Autodesk Inventor part; units mm, degrees
ref_plane "b_s_XY" through (0, 38, 5) normal (0, 1, 0) x (1, 0, 0)
ref_plane "b_s_YZ" through (0, 38, 5) normal (1, 0, 0) x (0, 0, -1)
ref_plane "b_s_ZX" through (0, 38, 5) normal (0, 0, -1) x (0, 1, 0)
sketch "Sketch_9" plane through (0, 0, 0) normal (0, 0, 1) x (1, 0, 0)
  line L0 (-15, 5) -> (-15, 0)
  line L1 (-15, 0) -> (15, 0)
  line L2 (15, 0) -> (15, 5)
  arc A0 (15, 5) -> (14, 6) centre (14, 5) ccw
  line L3 (14, 6) -> (-14, 6)
  arc A1 (-14, 6) -> (-15, 5) centre (-14, 5) ccw
sketch "Sketch_10" plane through (0, 0, 0) normal (0, 1, 0) x (-1, 0, 0)
  line L0 (15, 1) -> (15, 9)
  arc A0 (15, 9) -> (14, 10) centre (14, 9) ccw
  line L1 (14, 10) -> (-14, 10)
  arc A1 (-14, 10) -> (-15, 9) centre (-14, 9) ccw
  line L2 (-15, 9) -> (-15, 1)
  arc A2 (-15, 1) -> (-14, 0) centre (-14, 1) ccw
  line L3 (-14, 0) -> (14, 0)
  arc A3 (14, 0) -> (15, 1) centre (14, 1) ccw
extrude "Extrusion1" add sketch "Sketch_9" along normal blind 20
extrude "Extrusion2" add sketch "Sketch_10" along normal blind 38
sketch "Sketch_5" plane through (0, 0, 0) normal (0, 0, 1) x (1, 0, 0)
  arc A0 (-14, 38) -> (-15, 37) centre (-14, 37) ccw
  line L0 (-14, 38) -> (14, 38)
  arc A1 (15, 37) -> (14, 38) centre (14, 37) ccw
  line L1 (15, 37) -> (15, 76)
  line L2 (15, 76) -> (-15, 76)
  line L3 (-15, 76) -> (-15, 37)
extrude "Extrusion3" cut sketch "Sketch_5" along normal blind 10
sketch "Sketch_7" plane through (0, 0, 0) normal (1, 0, 0) x (0, 1, 0)
  line L0 (25, 0) -> (25, 10)
  line L1 (25, 10) -> (34, 10)
  line L2 (34, 10) -> (33, 9)
  line L3 (33, 9) -> (33, 1)
  line L4 (33, 1) -> (34, 0)
  line L5 (34, 0) -> (25, 0)
  line L6 (25, 0) -> (25, 10)
revolve "Revolution1" cut sketch "Sketch_7" angle 360 about axis through (0, 25, 0) along (0, 0, -1)
sketch "Sketch_1" plane through (0, 0, 5) normal (0, 0, 1) x (1, 0, 0)
  line L0 (0, 25) -> (0, 38)
  line L1 (0, 38) -> (2, 38)
  line L2 (2, 38) -> (1.621, 37.621)
  line L3 (1.621, 37.621) -> (1.621, 33)
  line L4 (1.621, 33) -> (2, 32.621)
  line L5 (2, 32.621) -> (2, 25)
  line L6 (2, 25) -> (0, 25)
  line L7 (0, 25) -> (0, 38)
revolve "Revolution2" cut sketch "Sketch_1" angle 360 about axis through (0, 25, 5) along (0, -1, 0)
thread "Thread1"
sketch "Sketch6" plane through (-14, 6, 20) normal (0, 1, 0) x (1, 0, 0)
  point P0 (7.5, 5)
hole "Hole1" at (-6.5, 6, 15) direction (0, -1, 0) diameter 5.5 depth 6 countersink diameter 6.5 countersink angle 90
sketch "Sketch7" plane through (-14, 6, 20) normal (0, 1, 0) x (1, 0, 0)
  point P0 (20.5, 5)
hole "Hole2" at (6.5, 6, 15) direction (0, -1, 0) diameter 5.5 depth 6 countersink diameter 6.5 countersink angle 90
sketch "Sketch_4" plane through (0, 0, 0) normal (0, 1, 0) x (-1, 0, 0)
  line L0 (30, -10) -> (30, 30)
  line L1 (30, 30) -> (-30, 30)
  line L2 (-30, 30) -> (-30, -10)
  line L3 (-30, -10) -> (30, -10)
  line L4 (15, 1) -> (15, 19)
  arc A0 (15, 19) -> (14, 20) centre (14, 19) ccw
  line L5 (14, 20) -> (-14, 20)
  arc A1 (-14, 20) -> (-15, 19) centre (-14, 19) ccw
  line L6 (-15, 19) -> (-15, 1)
  arc A2 (-15, 1) -> (-14, 0) centre (-14, 1) ccw
  line L7 (-14, 0) -> (14, 0)
  arc A3 (14, 0) -> (15, 1) centre (14, 1) ccw
extrude "Extrusion4" cut sketch "Sketch_4" along normal blind 38
sketch "Sketch_8" plane through (0, 0, 0) normal (0, 0, 1) x (1, 0, 0)
  line L0 (-7, 10) -> (-7, 2)
  line L1 (-7, 2) -> (7, 2)
  line L2 (7, 2) -> (7, 10)
  line L3 (7, 10) -> (-7, 10)
extrude "Extrusion5" cut sketch "Sketch_8" along normal blind 0.8
sketch "Sketch_6" plane through (0, 0, 0) normal (1, 0, 0) x (0, 1, 0)
  line L0 (57, 30) -> (-19, 30)
  line L1 (-19, 30) -> (-19, -10)
  line L2 (-19, -10) -> (57, -10)
  line L3 (57, -10) -> (57, 30)
  line L4 (5, 20) -> (0, 20)
  line L5 (0, 20) -> (0, 0)
  line L6 (0, 0) -> (37, 0)
  arc A0 (37, 0) -> (38, 1) centre (37, 1) ccw
  line L7 (38, 1) -> (38, 9)
  arc A1 (38, 9) -> (37, 10) centre (37, 9) ccw
  line L8 (37, 10) -> (6, 10)
  line L9 (6, 10) -> (6, 19)
  arc A2 (6, 19) -> (5, 20) centre (5, 19) ccw
extrude "Extrusion6" cut sketch "Sketch_6" along normal mid plane 30
sketch "Sketch_11" plane through (0, 0, 0) normal (1, 0, 0) x (0, 1, 0)
  line L0 (6, 11) -> (3, 11)
  line L1 (3, 11) -> (3, 5)
  line L2 (3, 5) -> (7, 5)
  line L3 (7, 5) -> (7, 10)
  arc A0 (6, 11) -> (7, 10) centre (7, 11) ccw
extrude "Extrusion7" add sketch "Sketch_11" along normal mid plane 28
ref_plane "b_s_XY" through (0, 38, 5) normal (0, 1, 0) x (1, 0, 0)
ref_plane "b_s_YZ" through (0, 38, 5) normal (1, 0, 0) x (0, 0, -1)
ref_plane "b_s_ZX" through (0, 38, 5) normal (0, 0, -1) x (0, 1, 0)
properties part number "SHKLMT16b"
The model under review builds one solid part; all positions refer to its coordinate system, in mm. A direction names the side the tool comes from. Coordinates: 2 decimals unless noted, no trailing zeros. Order: outer loops, then holes, each group sorted by start corner. A loop starts at its lowest first (then second) coordinate and runs counter-clockwise, first axis right, second up. Notation, with made-up numbers: (-33, 81.25) -> (-8, 81.25) arc R21 ccw to (-8, 87.25) -> close; hole circle Ø7 at (7, 0). An arc over 180 degrees is marked (long way). Answer in a Markdown table with one row per item.
(1) Insertion check: pin 1 (9 mm diameter, centred on x = -0.5, y = 6.5, fed in from -Z); pin 2 (5 mm diameter, centred on x = -6.5, z = 15, fed in from +Y); pin 3 (0.8 mm diameter, centred on y = 6.5, z = 10.5, fed in from +X); pin 4 (14 mm diameter, centred on x = 0, y = 17, fed in from +Z). Each pin has a flat end and moves straight along its axis. Give the tip position at first contact, or say it passes through.
Answers:
| item | result |
|---|---|
| pin 1 | z = 0 |
| pin 2 | through |
| pin 3 | x = 14 |
| pin 4 | z = 10 |
(2) Consider section D-D (z = 5). Write out the cut boundary in (x, y), plus the area to 3 significant figures.
Answers:
| item | result |
|---|---|
| outline | (-15, 0) -> (15, 0) -> (15, 37) arc R1 ccw to (14, 38) -> (2, 38) -> (1.62, 37.62) -> (1.62, 33) -> (1.83, 32.79) arc R8 cw (long way) to (-1.83, 32.79) -> (-1.62, 33) -> (-1.62, 37.62) -> (-2, 38) -> (-14, 38) arc R1 ccw to (-15, 37) -> close |
| area | 922 mm² |
(3) The part is to be moulded in two halves that separate along Y. For faces 4 (the cylindrical face through (14.715, 21.125, 9.699)), 5 (the cylindrical face through (-0.206, 37.699, 9.715)), 6 (the flat face through (0, 6, 0.8)), say which applies: +Y half, -Y half, draft (parallel to the pull), parting line (faces both ways), or undercut.
Answers:
| item | result |
|---|---|
| face 4 | draft |
| face 5 | +Y half |
| face 6 | undercut |
(4) Wall thickness on line 1 along X through (y, z) = (3.85, 15); line 2 along Z through (x, y) = (6.5, 1.65); line 3 along X through (y, z) = (25, 3.75): over which ranges is each line inside the solid? List them lowest first.
Answers:
| item | result |
|---|---|
| line 1 | -15 to -9.25, -3.75 to 3.75, 9.25 to 15 |
| line 2 | 0 to 12.25, 17.75 to 20 |
| line 3 | -15 to -8, 8 to 15 |
(5) Consider section A-A (y = 25). Write out the cut boundary in (x, z), plus the area to 3 significant figures.
Answers:
| item | result |
|---|---|
| outline | (-15, 1) arc R1 ccw to (-14, 0) -> (-9, 0) -> (-8, 1) -> (-8, 9) -> (-9, 10) -> (-14, 10) arc R1 ccw to (-15, 9) -> close; (8, 1) -> (9, 0) -> (14, 0) arc R1 ccw to (15, 1) -> (15, 9) arc R1 ccw to (14, 10) -> (9, 10) -> (8, 9) -> close |
| area | 137 mm² |
(6) Machinability: for faces 1 (the cylindrical face through (0.748, 35.278, 3.562)), 2 (the cylindrical face through (-4.827, 2.712, 12.818)), 3 (the flat face through (0, 15, 10)), which of the approach directions +Z, -Z, +X, -X, +Y, -Y give a long, thin tool a straight path to every point of the face, cutting with its end or side? Answer none if there is none.
Answers:
| item | result |
|---|---|
| face 1 | +Y |
| face 2 | +Y, -Y |
| face 3 | +Z, +X, -X, +Y |
(7) Consider section B-B (z = 15). Write out the cut boundary in (x, y), plus the area to 3 significant figures.
Answers:
| item | result |
|---|---|
| outline | (-15, 0) -> (-9.25, 0) -> (-9.25, 5.5) -> (-9.75, 6) -> (-14, 6) arc R1 ccw to (-15, 5) -> close; (-3.75, 0) -> (3.75, 0) -> (3.75, 5.5) -> (3.25, 6) -> (-3.25, 6) -> (-3.75, 5.5) -> close; (9.25, 0) -> (15, 0) -> (15, 5) arc R1 ccw to (14, 6) -> (9.75, 6) -> (9.25, 5.5) -> close |
| area | 113 mm² |
(8) Consider section C-C (x = 12.5). Write out the cut boundary in (y, z).
Answers:
| item | result |
|---|---|
| outline | (0, 0) -> (37, 0) arc R1 ccw to (38, 1) -> (38, 9) arc R1 ccw to (37, 10) -> (7, 10) arc R1 cw to (6, 11) -> (6, 19) arc R1 ccw to (5, 20) -> (0, 20) -> close |
